Design review of the part built by this model. Coordinates are the model's own, in mm. A direction names the side the tool comes from. Round coordinates to 2 decimals unless told otherwise and drop trailing zeros. Order: outer loops, then holes, each group sorted by start corner. A loop starts at its lowest first (then second) coordinate and runs counter-clockwise, first axis right, second up. Notation, with made-up numbers: (-17.5, -32) - (-6.5, -32) arc R13 cw to (-6.5, -27) - close; hole circle Ø11 at (41, 67.5). An arc over 180 degrees is marked (long way). Answer as a JSON object with one key per item and string values. Group by question number.
from build123d import *

# Parameters (mm, degrees)
CYLINDER001_R           = 1.1
CYLINDER001_DEPTH       = 15
CYLINDER001_PITCH_ANGLE = 90
BOX002_W                = 10
BOX002_H                = 6
BOX002_DEPTH            = 8
CYLINDER_R              = 4
CYLINDER_DEPTH          = 10
CYLINDER_PITCH_ANGLE    = 90
BOX001_W                = 6
BOX001_H                = 12
BOX001_DEPTH            = 19.5
BOX_W                   = 10
BOX_H                   = 12
BOX_DEPTH               = 23.5


with BuildPart() as cylinder001:
    # Cylinder001 → Cylinder001 (new body)
    with BuildSketch(Plane.XY):
        Circle(CYLINDER001_R)
    extrude(amount=CYLINDER001_DEPTH)


with BuildPart() as cylinder001_1:
    # Cylinder001 pitch: moved
    add(cylinder001.part.rotate(Axis((0, 0, 0), (0, 1, 0)), CYLINDER001_PITCH_ANGLE))


with BuildPart() as cylinder001_2:
    # Cylinder001 placement: moved
    add(cylinder001_1.part.moved(Location((7, 6, 11.75))))


with BuildPart() as cube002:
    # Box002 → Box002 (new body)
    with BuildSketch(Plane(origin=(10, 0, 7.75), x_dir=(1, 0, 0), z_dir=(0, 0, 1))):
        with Locations((5, 3)):
            Rectangle(BOX002_W, BOX002_H)
    extrude(amount=BOX002_DEPTH)


with BuildPart() as cylinder:
    # Cylinder → Cylinder (new body)
    with BuildSketch(Plane.XY):
        Circle(CYLINDER_R)
    extrude(amount=CYLINDER_DEPTH)


with BuildPart() as cylinder_1:
    # Cylinder pitch: moved
    add(cylinder.part.rotate(Axis((0, 0, 0), (0, 1, 0)), CYLINDER_PITCH_ANGLE))


with BuildPart() as cylinder_2:
    # Cylinder placement: moved
    add(cylinder_1.part.moved(Location((10, 6, 11.75))))


with BuildPart() as cube001:
    # Box001 → Box001 (new body)
    with BuildSketch(Plane(origin=(2, 0, 2), x_dir=(1, 0, 0), z_dir=(0, 0, 1))):
        with Locations((3, 6)):
            Rectangle(BOX001_W, BOX001_H)
    extrude(amount=BOX001_DEPTH)


with BuildPart() as cut001:
    # Box → Box (new body)
    with BuildSketch(Plane.XY):
        with Locations((5, 6)):
            Rectangle(BOX_W, BOX_H)
    extrude(amount=BOX_DEPTH)

    # Cut: cut Cube001
    add(cube001.part, mode=Mode.SUBTRACT)

    # Fusion: union Cylinder
    add(cylinder_2.part)

    # Fusion001: union Cube002
    add(cube002.part)

    # Cut001: cut Cylinder001
    add(cylinder001_2.part, mode=Mode.SUBTRACT)


solid = cut001.part
1. Take a section at B-B, the plane y = 3.5. Give the boundary of the cut face in (x, z), then the cut area to 3 significant figures.
2. Take a section at D-D, the plane z = 3.25. Give the boundary of the cut face in (x, y), then the cut area to 3 significant figures.
3. Tool access review of faces 4 (the flat face through (8, 4.6, 11.6)), 5 (the cylindrical face through (14.9, 10, 11.7)), 6 (the flat face through (15, 3, 15.75)), 7 (the flat face through (15, 3, 7.75)): name each direction out of +Z, -Z, +X, -X, +Y, -Y from which nothing blocks a thin tool from reaching the whole face with its end or side.
4. Mouldability with a two-part tool opening along Z and no side actions: class faces 1 (the cylindrical face through (13.92, 6.33, 10.7)), 2 (the flat face through (0, 6, 12)), 3 (the flat face through (5, 6, 23.5)) as pulls with the +Z half, pulls with the -Z half, needs draft (parallel to the pull), parting line crosses it, or undercut.
5. To check wall thickness, follow line 1 (Z direction, x = 14, y = 6); line 2 (X direction, y = 3.75, z = 6.25); line 3 (X direction, y = 7, z = 8.25). State the ranges of each line that lie inside material, in increasing order. Write a range as from..to.
6. Clearance check with flat-ended pins moving along their axes: P1, Ø1.8, axis at x = 15.5, y = 4.5, coming from the -Z side; P2, Ø1.5, axis at x = 2.5, z = 12.5, coming from the +Y side; P3, Ø1.5, axis at x = 13.5, y = 7.5, coming from the +Z side; P4, Ø3, axis at x = 16.5, y = 10, coming from the -Z side. State where each tip first meets the part, or that it passes through.
7. Take a section at A-A, the plane z = 11.75. Give the boundary of the cut face in (x, y), then the cut area to 3 significant figures.
8. Take a section at C-C, the plane x = 16.5. Give the boundary of the cut face in (y, z).
Response values:
{
 "1": {"outline": "(0, 0) - (10, 0) - (10, 7.75) - (20, 7.75) - (20, 15.75) - (10, 15.75) - (10, 23.5) - (0, 23.5) - close; hole (2, 2) - (8, 2) - (8, 21.5) - (2, 21.5) - close", "area": "198 mm2"},
 "2": {"outline": "(0, 0) - (2, 0) - (2, 12) - (0, 12) - close; (8, 0) - (10, 0) - (10, 12) - (8, 12) - close", "area": "48.0 mm2"},
 "3": {"face 4": "+Y, -Y", "face 5": "+X, +Y", "face 6": "+Z, +X, +Y, -Y", "face 7": "-Z, +X, +Y, -Y"},
 "4": {"face 1": "undercut", "face 2": "needs draft", "face 3": "pulls with the +Z half"},
 "5": {"line 1": "7.75..10.65, 12.85..15.75", "line 2": "0..2, 8..10", "line 3": "0..2, 8..20"},
 "6": {"P1": "z = 7.75", "P2": "y = 12", "P3": "z = 15.68", "P4": "z = 8.63"},
 "7": {"outline": "(0, 0) - (2, 0) - (2, 12) - (0, 12) - close; (8, 0) - (20, 0) - (20, 4.9) - (8, 4.9) - close; (8, 7.1) - (20, 7.1) - (20, 10) - (10, 10) - (10, 12) - (8, 12) - close", "area": "122 mm2"},
 "8": {"outline": "(0, 7.75) - (6, 7.75) arc R4 ccw to (6, 15.75) - (0, 15.75) - close; hole circle Ø2.2 at (6, 11.75)"}
}
